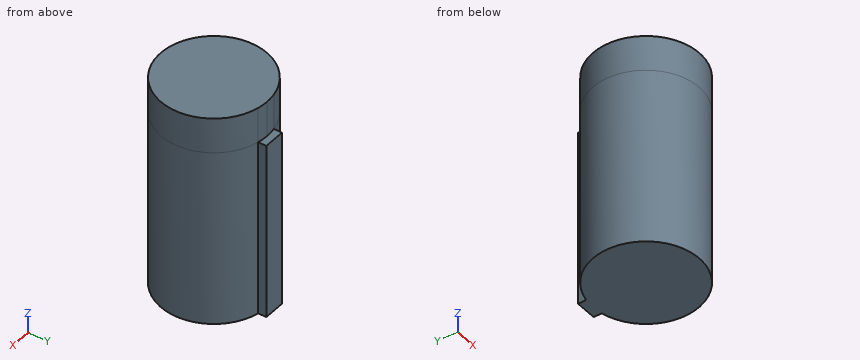
Solid Edge part; units mm, degrees
sketch "Sketch1" plane through (0, 0, 0) normal (0, 0, 1) x (1, 0, 0)
  circle A0 centre (0, -0.5) radius 7.5
  line L0 (1.5, 8) -> (-1.5, 8)
  line L1 (-1.5, 8) -> (-1.5, 6)
  line L2 (-1.5, 6) -> (1.5, 6)
  line L3 (1.5, 6) -> (1.5, 8)
extrude "Protrusion1" add sketch "Sketch1" along normal blind 30
sketch "Sketch2" plane through (0, 0, 30) normal (0, 0, 1) x (0, 1, 0)
  circle A0 centre (-0.5, 0) radius 9
  circle A1 centre (-0.5, 0) radius 7.5
extrude "ExtrudedCutout_3" cut sketch "Sketch2" against normal blind 5
properties material "Stainless steel"
Design review of the part built by this model. Coordinates are the model's own, in mm. Coordinates: 2 decimals unless noted, no trailing zeros. Order: outer loops, then holes, each group sorted by start corner. A loop starts at its lowest first (then second) coordinate and runs counter-clockwise, first axis right, second up. Notation, with made-up numbers: (52, 23) -> (65, 23) arc R26 cw to (65, 51) -> close; hole circle Ø6 at (-36.75, 56.25). An arc over 180 degrees is marked (long way). Use one line per item in the form item = value. Start each with the question number.
(1) Add section B-B on z = 5.5. State the section outline as (x, y) points, plus the area to 3 significant figures.
(2) Insertion check: pin 1 (8 mm diameter, centred on x = 5.5, z = 14.5, fed in from -Y); pin 2 (0.6 mm diameter, centred on y = 7.5, z = 14.5, fed in from +X). Each pin has a flat end and moves straight along its axis. Give the tip position at first contact, or say it passes through.
(3) Add section A-A on x = -1. State the section outline as (y, z) points.
(4) For probe 1 along X at (y, z) = (1.5, 18.25); probe 2 along Y at (x, z) = (0.25, 2.75); probe 3 along X at (y, z) = (2, 8.5), list the stretches that pass through material, from the lowest coordinate up.
(5) Add section C-C on y = -4. State the section outline as (x, z) points, plus the area to 3 significant figures.
Answer block:
q1.outline = (-1.5, 6.85) arc R7.5 ccw (long way) to (1.5, 6.85) -> (1.5, 8) -> (-1.5, 8) -> close
q1.area = 180 mm²
q2.pin_1 = -7.85
q2.pin_2 = 1.5
q3.outline = (-7.93, 0) -> (8, 0) -> (8, 25) -> (6.93, 25) -> (6.93, 30) -> (-7.93, 30) -> close
q4.probe_1 = -7.23 to 7.23
q4.probe_2 = -8 to 8
q4.probe_3 = -7.07 to 7.07
q5.outline = (-6.63, 0) -> (6.63, 0) -> (6.63, 30) -> (-6.63, 30) -> close
q5.area = 398 mm²
